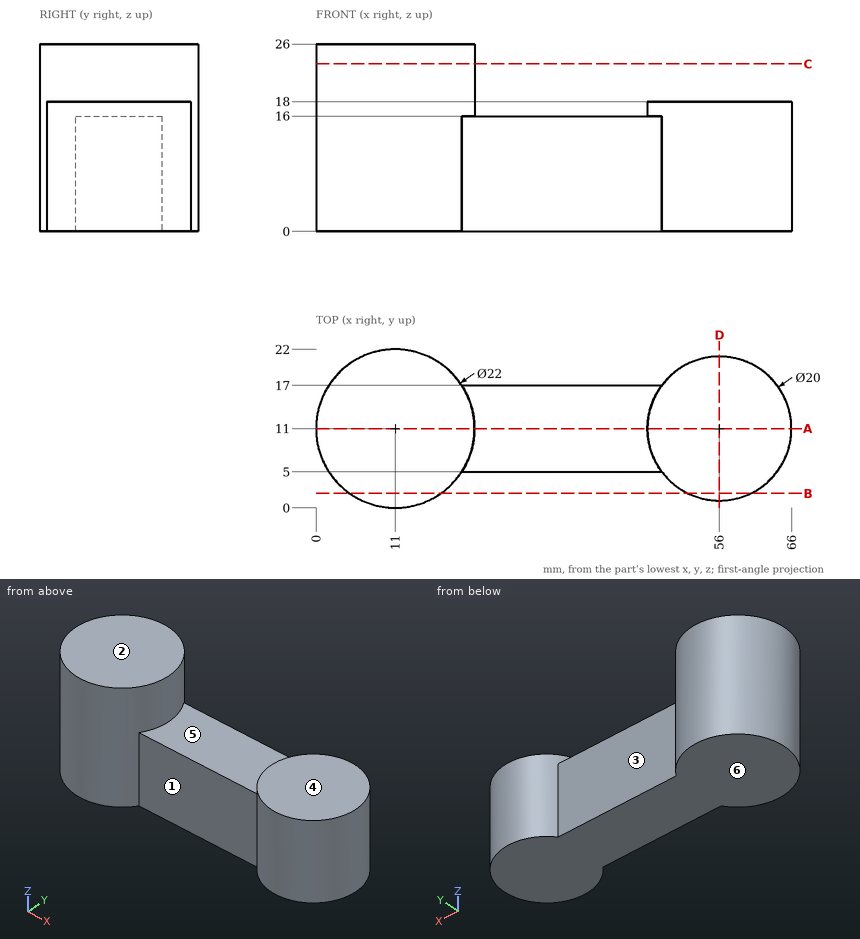
Verification items for this drawing (mm, ordinates from the low corner). A direction names the side the tool comes from. Give positions to 0.01 mm unless a question says otherwise; leave off trailing zeros. Loops run counter-clockwise (first coordinate to the right, second up) from the corner with the lowest first, then second, coordinate; pieces in that order, holes last. Notation, with made-up numbers: M 65,44 L 73,44 A19 ccw 73,81 Z; hole C 42.25,41.5 d5. An arc over 180 degrees is marked long. Answer as a JSON object with one key per item and string values. Group by question number.
Item 1: Sectioned sample at C-C on z = 23.25. Record the boundary of the cut face in (x, y), plus the area to 3 significant figures.
Item 2: Sectioned sample at D-D on x = 56. Record the boundary of the cut face in (y, z).
Item 3: Access from +Z, -Z, +X, -X, +Y, -Y to the whole of each face (thin tool, end or side, straight path). Record for the marked faces 1, 2, 3 and 4.
Item 4: Sectioned sample at A-A on y = 11. Record the boundary of the cut face in (x, z).
Item 5: Sectioned sample at B-B on y = 2. Record the boundary of the cut face in (x, z).
Item 6: Material ranges on L1, parallel to X at y = 10.75, z = 24.75; L2, parallel to Z at x = 28, y = 7.25; L3, parallel to Y at x = 25, z = 8.5, recorded low to high.
Item 7: Gauge pin test, flat ends, axial feed: pin 1 (1.5 mm diameter, centred on x = 47, y = 11.5, fed in from +Z); pin 2 (1.5 mm diameter, centred on x = 34, z = 13, fed in from -Y); pin 3 (2 mm diameter, centred on x = 14.5, z = 20, fed in from +Y). Record the tip position at first contact, or that the pin passes through.
Item 8: Mould release check, pull along X, two halves, no side actions. Record for the marked faces 5 and 6: pulls with the +X half, pulls with the -X half, needs draft (parallel to the pull), parting line crosses it, or undercut.
Findings below:
{
 "1": {"outline": "C 11,11 d22", "area": "380 mm2"},
 "2": {"outline": "M 1,0 L 21,0 L 21,18 L 1,18 Z"},
 "3": {"face 1": "+Z, -Z, -Y", "face 2": "+Z, +X, -X, +Y, -Y", "face 3": "+Z, -Z, +Y", "face 4": "+Z, +X, +Y, -Y"},
 "4": {"outline": "M 0,0 L 66,0 L 66,18 L 46,18 L 46,16 L 22,16 L 22,26 L 0,26 Z"},
 "5": {"outline": "M 4.68,0 L 17.32,0 L 17.32,26 L 4.68,26 Z; M 51.64,0 L 60.36,0 L 60.36,18 L 51.64,18 Z"},
 "6": {"L1": "0 to 22", "L2": "0 to 16", "L3": "5 to 17"},
 "7": {"pin 1": "z = 18", "pin 2": "y = 5", "pin 3": "y = 21.71"},
 "8": {"face 5": "undercut", "face 6": "needs draft"}
}
